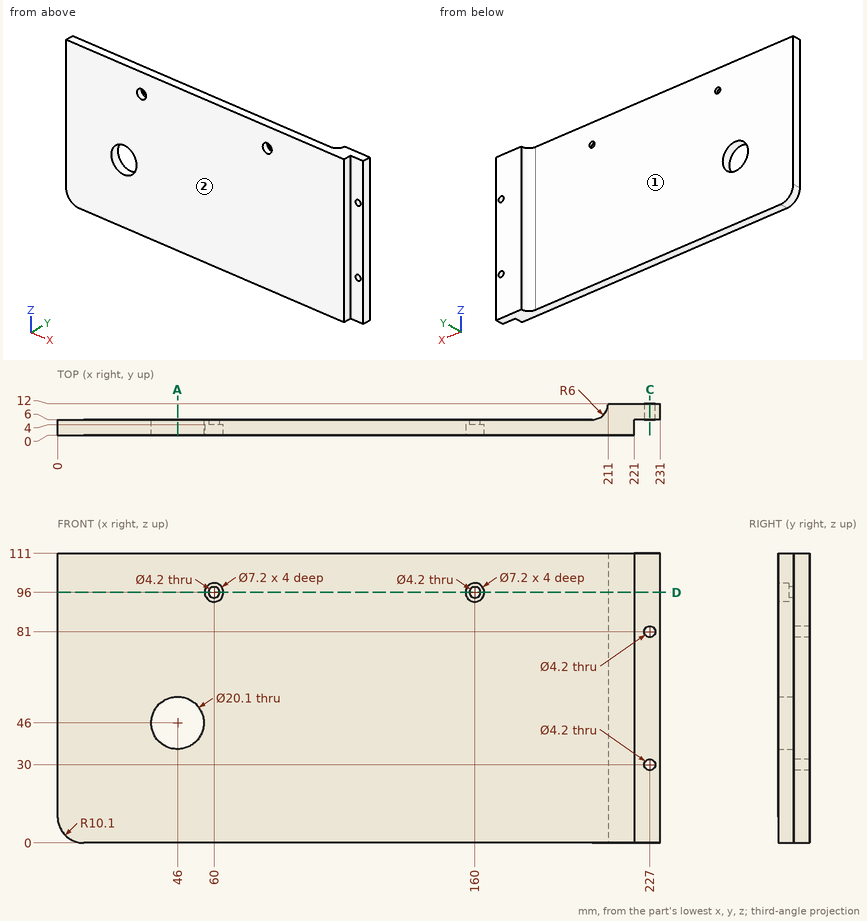
Answer from the drawing. Dimensions are ordinates in mm from the lowest x, y and z of the part. A direction names the side the tool comes from. Coordinates: 2 decimals unless noted, no trailing zeros. Write each loop counter-clockwise with the first axis right and the second up, starting at its lowest first coordinate (ties: lowest second). Pieces come first, ordered by that corner, then holes. Notation, with made-up numbers: (86, -21) - (126, -21) arc R18 ccw to (126, 10) - close; hole circle Ø9 at (53, 22). An arc over 180 degrees is marked (long way). Return JSON: item names as keys, results as strings.
1. The part is cut by section A-A on x = 46. Determine the outline of the cut face in (y, z).
Final values:
{"outline": "(0, 0) - (6, 0) - (6, 35.95) - (0, 35.95) - close; (0, 56.05) - (6, 56.05) - (6, 111) - (0, 111) - close"}
2. Each of these flat-tipped pins is pushed along its axis until it touches: pin 1 Ø3.5 at (x, z) = (227, 30) entering from -Y; pin 2 Ø3 at (x, z) = (226, 80) entering from -Y; pin 3 Ø10 at (x, z) = (61.5, 91) entering from +Y; pin 4 Ø5 at (x, z) = (60, 96) entering from -Y. Where does it stop, or does it pass through?
Final values:
{"pin 1": "through", "pin 2": "y = 6", "pin 3": "y = 6", "pin 4": "y = 4"}
3. The part is cut by section C-C on x = 227. Determine the outline of the cut face in (y, z).
Final values:
{"outline": "(6, 0) - (12, 0) - (12, 27.9) - (6, 27.9) - close; (6, 32.1) - (12, 32.1) - (12, 78.9) - (6, 78.9) - close; (6, 83.1) - (12, 83.1) - (12, 111) - (6, 111) - close"}
4. The part is cut by section D-D on z = 96. Count the separate pieces of the cut face and the enclosed holes in it, then the cut area to 3 significant figures.
Final values:
{"separate pieces": "3", "enclosed holes": "0", "area": "1,380 mm^2"}
5. Consider line 1 along Z through (x, y) = (227, 9.25); line 2 along Z through (x, y) = (60, 2); line 3 along Z through (x, y) = (160, 5.2). Determine where each line is inside the solid, lowest interval first.
Final values:
{"line 1": "0 to 27.9, 32.1 to 78.9, 83.1 to 111", "line 2": "0 to 92.4, 99.6 to 111", "line 3": "0 to 93.9, 98.1 to 111"}
6. Which of the six approach directions +Z, -Z, +X, -X, +Y, -Y give full straight-line access (tool end or side, diameter ignored) to the marked faces 1 and 2?
Final values:
{"face 1": "+Z, -Z, -X, +Y", "face 2": "+Z, -Z, +X, -X, -Y"}
